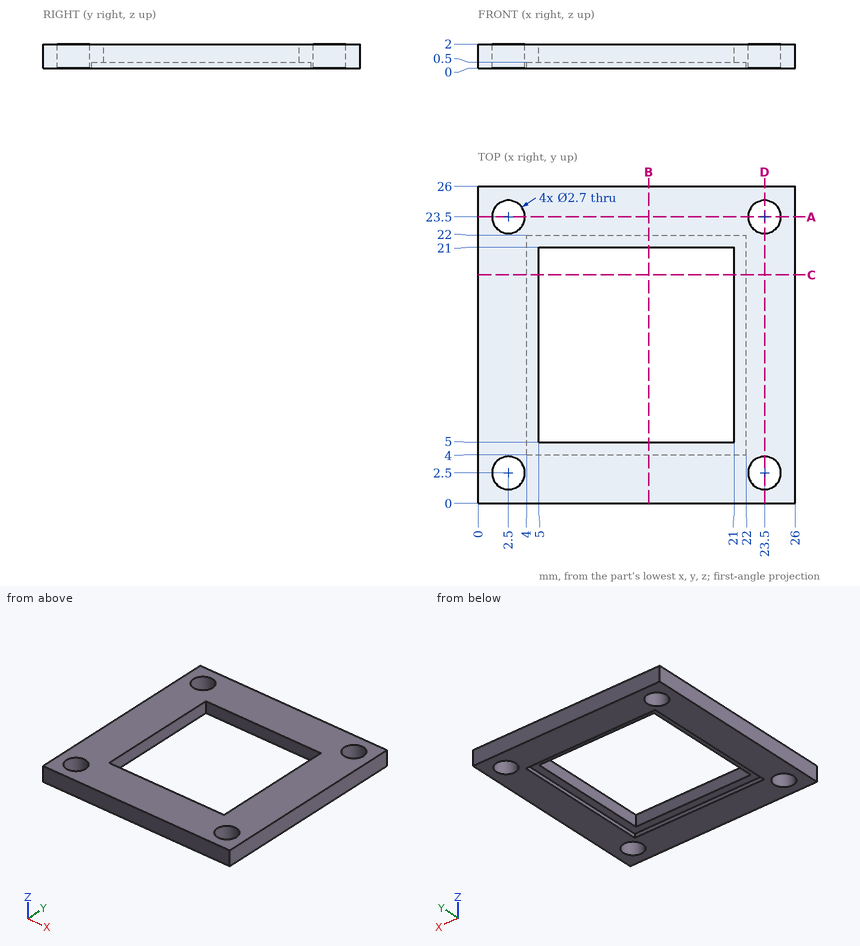
For this review, use the dimensioned drawing (mm, ordinates from the lowest corner) and the shaded views. Coordinates: 2 decimals unless noted, no trailing zeros. Loops run counter-clockwise (first coordinate to the right, second up) from the corner with the lowest first, then second, coordinate; pieces in that order, holes last. Notation, with made-up numbers: (20.25, 78) - (29.25, 78) arc R19 ccw to (29.25, 83) - close; hole circle Ø7 at (57.25, 10). An arc over 180 degrees is marked (long way). Use one line per item in the form item = value. Start each with the question number.
1) Take a section at B-B (x = 14). State the section outline as (y, z) points.
2) Take a section at A-A (y = 23.5). State the section outline as (x, z) points, plus the area to 3 significant figures.
3) To check wall thickness, follow probe 1 along Y at (x, z) = (23.5, 0.9); probe 2 along Y at (x, z) = (9.5, 1.5). State the ranges of each line that lie inside material, in increasing order. Write a range as from..to.
From the geometry:
q1.outline = (0, 0) - (4, 0) - (4, 0.5) - (5, 0.5) - (5, 2) - (0, 2) - close; (21, 0.5) - (22, 0.5) - (22, 0) - (26, 0) - (26, 2) - (21, 2) - close
q2.outline = (0, 0) - (1.15, 0) - (1.15, 2) - (0, 2) - close; (3.85, 0) - (22.15, 0) - (22.15, 2) - (3.85, 2) - close; (24.85, 0) - (26, 0) - (26, 2) - (24.85, 2) - close
q2.area = 41.2 mm2
q3.probe_1 = 0..1.15, 3.85..22.15, 24.85..26
q3.probe_2 = 0..5, 21..26
